Model file for the job. Use its own axes, mm. A direction names the side the tool comes from. Coordinates: 2 decimals unless noted, no trailing zeros. Write each loop counter-clockwise with the first axis right and the second up, starting at its lowest first coordinate (ties: lowest second). Pieces come first, ordered by that corner, then holes. Notation, with made-up numbers: M -21.75,-21 L -10.75,-21 A8 cw -10.75,-6 Z; hole C 23.25,45 d8. An arc over 180 degrees is marked long. Put each result on its own line as item: value. Start each with the question number.
Q1. Drop flat-ended pins along their axis: pin 1 (2 mm diameter, centred on x = -1, y = -32.5, fed in from -Z); pin 2 (3 mm diameter, centred on x = 8.5, y = 28, fed in from -Z); pin 3 (3.5 mm diameter, centred on x = 31.75, y = 0, fed in from -Z); pin 4 (6 mm diameter, centred on y = -6, z = 15.5, fed in from +X). Give the stop position or say it passes through.
Q2. Cut at C-C (z = 17.25). Write the cut outline in (x, y).
Q3. Which spindle directions (+Z, -Z, +X, -X, +Y, -Y) get a long thin tool onto all of the face, cutting with end or side? Do faces 4 (the flat face through (-8, 8, 19.05)), 5 (the flat face through (2, -31, 16.205)), 6 (the cylindrical face through (-0.396, 29.965, 17.648)). Say none if no direction does.
Q4. Cut at A-A (x = 0). Give the number of separate pieces and of enclosed holes in the cut face, then the cut area to 3 significant figures.
Q5. Cut at D-D (z = 6.25). Write the cut outline in (x, y), then the cut area to 3 significant figures.
Q6. Pull direction X, two halves, no side cores. Call faces 1 (the flat face through (16, -1, 12.7)), 2 (the cylindrical face through (12, -4, 7)), 3 (the flat face through (2, 33, 16.205)): pulls with the +X half, pulls with the -X half, needs draft (parallel to the pull), parting line crosses it, or undercut.
Q7. Drill centre lines: line 1 along Y through (x, z) = (0, 14.15); line 2 along Y through (x, z) = (0, 16.85); line 3 along X through (y, z) = (-1.5, 16). Where is each one in solid material? Low to high.
```python
from build123d import *

# Parameters (mm, degrees)
CBORE_FOR_6_SOCKET_HEAD_CAP_SCREW1_D           = 3.6576
CBORE_FOR_6_SOCKET_HEAD_CAP_SCREW1_CBORE_D     = 7.14502
CBORE_FOR_6_SOCKET_HEAD_CAP_SCREW1_CBORE_DEPTH = 3.5052
CHAMFER1_SIZE                                  = 0.508


with BuildPart() as part:
    # Sketch1 → Revolve1 (revolve)
    with BuildSketch(Plane(origin=(0, 0, 0), x_dir=(0, 0, -1), z_dir=(1, 0, 0)), mode=Mode.PRIVATE) as revolve1_sk:
        Polygon((-22.225, 0), (-22.225, 9.5123), (-19.05, 9.5123), (-19.05, 37.846), (-12.7, 37.846), (-12.7, 12.6492), (0, 12.6492), (0, 0), align=None)
    revolve(revolve1_sk.sketch.rotate(Axis((0, 0, 22.225), (0, 0, -1)), 90), axis=Axis((0, 0, 22.225), (0, 0, -1)))

    # CBORE for #6 Socket Head Cap Screw1 (through all)
    with Locations(Plane(origin=(0, 0, 12.7), x_dir=(-1, 0, 0), z_dir=(0, 0, -1))):
        with Locations((-31.75, 0), (0, 31.75), (31.75, 0), (0, -31.75)):
            CounterBoreHole(CBORE_FOR_6_SOCKET_HEAD_CAP_SCREW1_D / 2, CBORE_FOR_6_SOCKET_HEAD_CAP_SCREW1_CBORE_D / 2, CBORE_FOR_6_SOCKET_HEAD_CAP_SCREW1_CBORE_DEPTH)

    # Chamfer1
    chamfer1_edges = [part.edges().sort_by_distance(p)[0] for p in [
        (-12.6492, 0, 0),
        (-37.846, 0, 12.7),
    ]]
    chamfer(chamfer1_edges, length=CHAMFER1_SIZE)


solid = part.part
```
Computed values:
1. pin 1: z = 16.21
1. pin 2: z = 12.7
1. pin 3: through
1. pin 4: x = 37.73
2. outline: C 0,0 d75.69; hole C -31.75,0 d3.66; hole C 0,-31.75 d3.66; hole C 0,31.75 d3.66; hole C 31.75,0 d3.66
3. face 4: +Z
3. face 5: -Z
3. face 6: +Z, -Z
4. separate pieces: 3
4. enclosed holes: 0
4. area: 791 mm2
5. outline: C 0,0 d25.3
5. area: 503 mm2
6. face 1: needs draft
6. face 2: parting line crosses it
6. face 3: undercut
7. line 1: -37.85 to -35.32, -28.18 to 28.18, 35.32 to 37.85
7. line 2: -37.85 to -33.58, -29.92 to 29.92, 33.58 to 37.85
7. line 3: -37.82 to -34.99, -28.51 to 28.51, 34.99 to 37.82
